Verification items for the finished model (mm, model axes). A direction names the side the tool comes from. Round coordinates to 2 decimals unless told otherwise and drop trailing zeros. Order: outer loops, then holes, each group sorted by start corner. A loop starts at its lowest first (then second) coordinate and runs counter-clockwise, first axis right, second up. Notation, with made-up numbers: (-37.75, -39.5) -> (-33.75, -39.5) arc R22 cw to (-33.75, -0.5) -> close; hole circle Ø1 at (-9.75, 16.25). An arc over 180 degrees is marked (long way). Put each result on its own line as item: value.
from build123d import *

# Parameters (mm, degrees)
F1_DEPTH  = 2082.8
F3_DEPTH  = 204.7885
F5_DEPTH  = 996.95
F7_DEPTH  = 204.7885
F10_DEPTH = 914.4
F12_DEPTH = 0.79475
F13_W     = 6.35
F13_H     = 100.0125
F14_DEPTH = 2082.801


with BuildPart() as f1:
    # F0 (on Top) → F1 (new body)
    with BuildSketch(Plane.XY):
        Polygon((-41.275, 46.0375), (-41.275, 0), (0, 0), (0, 0.79375), (-34.925, 0.79375), (-34.925, 52.3875), (-47.625, 52.3875), (-47.625, 152.4), (-34.925, 152.4), (-34.925, 203.99375), (0, 203.99375), (0, 204.7875), (-41.275, 204.7875), (-41.275, 158.75), (-53.975, 158.75), (-53.975, 46.0375), align=None)
    extrude(amount=F1_DEPTH)


with BuildPart() as f1b:
    # F0 (on Top) → F1, piece 2 (new body)
    with BuildSketch(Plane.XY):
        Polygon((-996.95, 0.79375), (-996.95, 0), (-955.675, 0), (-955.675, 46.0375), (-942.975, 46.0375), (-942.975, 158.75), (-955.675, 158.75), (-955.675, 204.7875), (-996.95, 204.7875), (-996.95, 203.99375), (-962.025, 203.99375), (-962.025, 152.4), (-949.325, 152.4), (-949.325, 52.3875), (-962.025, 52.3875), (-962.025, 0.79375), align=None)
    extrude(amount=F1_DEPTH)


with BuildPart() as f3_tool:
    # F2 (on Front) → F3 (new body, through all)
    with BuildSketch(Plane.XZ):
        Polygon((0, 2082.8), (-996.95, 2082.8), (-498.475, 1584.325), align=None)
    extrude(amount=-F3_DEPTH)


with BuildPart() as f1_1:
    add(f1.part)

    # F3: cut by f3_tool
    add(f3_tool.part, mode=Mode.SUBTRACT)


with BuildPart() as f1b_1:
    add(f1b.part)

    # F3: cut by f3_tool
    add(f3_tool.part, mode=Mode.SUBTRACT)


with BuildPart() as f5:
    # F4 (on Right) → F5 (new body, through all)
    with BuildSketch(Plane.YZ):
        Polygon((158.75, 2041.525), (204.7875, 2041.525), (204.7875, 2082.8), (203.99375, 2082.8), (203.99375, 2047.875), (152.4, 2047.875), (152.4, 2035.175), (52.3875, 2035.175), (52.3875, 2047.875), (0.79375, 2047.875), (0.79375, 2082.8), (0, 2082.8), (0, 2041.525), (46.0375, 2041.525), (46.0375, 2028.825), (158.75, 2028.825), align=None)
    extrude(amount=-F5_DEPTH)

    # F6 (on Front) → F7 (cut, through all)
    with BuildSketch(Plane.XZ):
        Polygon((0, 2082.8), (-498.475, 1584.325), (304.8, 1584.325), (304.8, 2082.8), align=None)
        Polygon((-498.475, 1584.325), (-996.95, 2082.8), (-1301.75, 2082.8), (-1301.75, 1584.325), align=None)
    extrude(amount=-F7_DEPTH, mode=Mode.SUBTRACT)


with BuildPart() as f1_2:
    add(f1_1.part)

    # F8: union F1b, F5
    add(f1b_1.part)
    add(f5.part)

    # F9 (on face) → F10 (join, through all)
    with BuildSketch(Plane(origin=(-41.275, 0, 0), x_dir=(0, -1, 0), z_dir=(-1, 0, 0))):
        Polygon((-203.99375, 0), (-102.39375, 0), (-0.79375, 0), (-26.19375, 12.7), (-102.39375, 12.7), (-178.59375, 12.7), align=None)
    extrude(amount=F10_DEPTH)

    # F11 (on face) → F12 (cut, through all)
    with BuildSketch(Plane(origin=(0, 0.79375, 0), x_dir=(-1, 0, 0), z_dir=(0, 1, 0))):
        Polygon((34.9250000001, 2047.875), (962.025, 2047.875), (962.025, 0), (996.95, 0), (996.95, 2082.8), (1e-10, 2082.8), (0, 0), (34.925, 0), align=None)
    extrude(amount=-F12_DEPTH, mode=Mode.SUBTRACT)

    # F13 (on Top) → F14 (cut, through all)
    with BuildSketch(Plane.XY):
        with Locations((-44.45, 102.39375)):
            Rectangle(F13_W, F13_H)
        with Locations((-952.5, 102.39375)):
            Rectangle(F13_W, F13_H)
    extrude(amount=F14_DEPTH, mode=Mode.SUBTRACT)


solid = f1_2.part
Item 1: Material ranges on L1, parallel to X at y = 68.5, z = 1819 (3 decimals); L2, parallel to Z at x = -546.5, y = 26 (3 decimals); L3, parallel to Z at x = -863, y = 96 (3 decimals), recorded low to high. Write a range as [from, to].
Check sheet entries:
L1: x = [-949.325, -942.975], [-53.975, -47.625]
L2: z = [0, 12.603], [2041.525, 2047.875]
L3: z = [0, 12.7], [2028.825, 2035.175]
Item 2: Release check for a two-part mould opening along Y. For faces 4 (the flat face through (-949.325, 102, 1003)), 5 (the flat face through (-955.675, 181, 1006)) record: +Y half, -Y half, draft (parallel to the pull), parting line (faces both ways), or undercut.
Check sheet entries:
face 4: undercut
face 5: draft
Item 3: Tool access check on faces 1 (the flat face through (-34.925, 178, 1010)), 2 (the flat face through (-962.025, 27, 1038)), 3 (the flat face through (-492, 181, 2041.525)). Record the directions out of +Z, -Z, +X, -X, +Y, -Y that give a thin tool (end or side, any length) a straight path to the whole face; none if there is none.
Check sheet entries:
face 1: +Z, -Z, +X, -Y
face 2: +Z, -Z, -X, -Y
face 3: +Y
Item 4: Gauge pin test, flat ends, axial feed: pin 1 Ø5 at (y, z) = (79, 224) entering from -X (3 decimals); pin 2 Ø3 at (y, z) = (160, 1472) entering from +X (3 decimals). Record the tip position at first contact, or that the pin passes through.
Check sheet entries:
pin 1: stops at x = -949.325
pin 2: stops at x = -34.925
Item 5: Section check C-C on y = 127. Record the boundary of the cut face in (x, z) (3 decimals), then the cut area to 3 significant figures.
Check sheet entries:
outline: (-949.325, 0) -> (-47.625, 0) -> (-47.625, 2035.175) -> (-949.325, 2035.175) -> close; hole (-942.975, 12.7) -> (-53.975, 12.7) -> (-53.975, 2028.825) -> (-942.975, 2028.825) -> close
area: 42,800 mm^2
